```python
from build123d import *

# Parameters (mm, degrees)
BOX044_W          = 50
BOX044_H          = 20
BOX044_DEPTH      = 30
BOX_W             = 10
BOX_H             = 10
BOX_DEPTH         = 30
CYLINDER011_R     = 2
CYLINDER011_DEPTH = 24
CYLINDER009_R     = 2
CYLINDER009_DEPTH = 24
CYLINDER008_R     = 2
CYLINDER008_DEPTH = 24
BOX001_W          = 20
BOX001_H          = 33
BOX001_DEPTH      = 3


with BuildPart() as cube040:
    # Box044 → Box044 (new body)
    with BuildSketch(Plane(origin=(-25, -32, -1), x_dir=(1, 0, 0), z_dir=(0, 0, 1))):
        with Locations((25, 10)):
            Rectangle(BOX044_W, BOX044_H)
    extrude(amount=BOX044_DEPTH)


with BuildPart() as cube:
    # Box → Box (new body)
    with BuildSketch(Plane(origin=(-5, 2, -1), x_dir=(1, 0, 0), z_dir=(0, 0, 1))):
        with Locations((5, 5)):
            Rectangle(BOX_W, BOX_H)
    extrude(amount=BOX_DEPTH)


with BuildPart() as cylinder007:
    # Cylinder011 → Cylinder011 (new body)
    with BuildSketch(Plane(origin=(-10, -13, 4.3), x_dir=(0, 0, -1), z_dir=(1, 0, 0))):
        Circle(CYLINDER011_R)
    extrude(amount=CYLINDER011_DEPTH)


with BuildPart() as cylinder005:
    # Cylinder009 → Cylinder009 (new body)
    with BuildSketch(Plane(origin=(-10, -11, -1.3), x_dir=(0, 0, -1), z_dir=(1, 0, 0))):
        Circle(CYLINDER009_R)
    extrude(amount=CYLINDER009_DEPTH)


with BuildPart() as cylinder004:
    # Cylinder008 → Cylinder008 (new body)
    with BuildSketch(Plane(origin=(-10, 11, -1.3), x_dir=(0, 0, -1), z_dir=(1, 0, 0))):
        Circle(CYLINDER008_R)
    extrude(amount=CYLINDER008_DEPTH)


with BuildPart() as paste_extruder_charger:
    # Box001 → Box001 (new body)
    with BuildSketch(Plane(origin=(-8.25, -16.5, 0), x_dir=(1, 0, 0), z_dir=(0, 0, 1))):
        with Locations((10, 16.5)):
            Rectangle(BOX001_W, BOX001_H)
    extrude(amount=BOX001_DEPTH)

    # Cut001: cut Cylinder004
    add(cylinder004.part, mode=Mode.SUBTRACT)

    # Cut002: cut Cylinder005
    add(cylinder005.part, mode=Mode.SUBTRACT)

    # Cut003: cut Cylinder007
    add(cylinder007.part, mode=Mode.SUBTRACT)

    # Cut063: cut Cube
    add(cube.part, mode=Mode.SUBTRACT)

    # Cut062: cut Cube040
    add(cube040.part, mode=Mode.SUBTRACT)


with BuildPart() as paste_extruder_charger_1:
    # Cut062 placement: moved
    add(paste_extruder_charger.part.moved(Location((0, 58, 0))))


solid = paste_extruder_charger_1.part
```
For this review, take the finished solid that the model builds, in its own axes (mm). A direction names the side the tool comes from. Round coordinates to 2 decimals unless told otherwise and drop trailing zeros. Write each loop counter-clockwise with the first axis right and the second up, starting at its lowest first coordinate (ties: lowest second). Pieces come first, ordered by that corner, then holes. Notation, with made-up numbers: (88.5, 3) -> (113.5, 3) arc R23 ccw to (113.5, 12) -> close; hole circle Ø5 at (66, 26). An arc over 180 degrees is marked (long way). Use one line per item in the form item = value.
1) Mouldability with a two-part tool opening along X and no side actions: class faces 1 (the flat face through (2, 74.5, 1)), 2 (the flat face through (11.75, 60, 1)), 3 (the flat face through (-5, 65, 1)) as +X half, -X half, draft (parallel to the pull), parting line (faces both ways), or undercut.
Found:
face_1 = draft
face_2 = +X half
face_3 = undercut
2) Take a section at A-A, the plane x = 1. Write out the cut boundary in (y, z), and give its area (3 significant figures).
Found:
outline = (46, 0.43) arc R2 cw to (48.52, 0) -> (60, 0) -> (60, 3) -> (46.52, 3) arc R2 cw to (46, 2.57) -> close; (70, 0.43) arc R2 cw to (70.52, 0) -> (74.5, 0) -> (74.5, 3) -> (70, 3) -> close
area = 53.9 mm2
3) To check wall thickness, follow L1, parallel to Y at x = 3.5, z = 0.8; L2, parallel to X at y = 63, z = 0.95; L3, parallel to Y at x = 3, z = 2.6. State the ranges of each line that lie inside material, in increasing order. Write a range as from..to.
Found:
L1 = 46..60, 70..74.5
L2 = -8.25..-5, 5..11.75
L3 = 46.05..60, 70..74.5
4) Take a section at B-B, the plane y = 60.5. Write out the cut boundary in (x, z).
Found:
outline = (-8.25, 0) -> (-5, 0) -> (-5, 3) -> (-8.25, 3) -> close; (5, 0) -> (11.75, 0) -> (11.75, 3) -> (5, 3) -> close
5) Take a section at D-D, the plane x = 7.5. Write out the cut boundary in (y, z), and give its area (3 significant figures).
Found:
outline = (46, 0.43) arc R2 cw to (48.52, 0) -> (67.48, 0) arc R2 cw to (70.52, 0) -> (74.5, 0) -> (74.5, 3) -> (46.52, 3) arc R2 cw to (46, 2.57) -> close
area = 82.5 mm2
6) Tool access review of faces 4 (the cylindrical face through (1.61, 47.357, 0.668)), 5 (the flat face through (5, 65, 1)): name each direction out of +Z, -Z, +X, -X, +Y, -Y from which nothing blocks a thin tool from reaching the whole face with its end or side.
Found:
face_4 = -Z, +X, -X
face_5 = +Z, -Z
7) Take a section at C-C, the plane z = 1.8. Write out the cut boundary in (x, y).
Found:
outline = (-8.25, 46) -> (11.75, 46) -> (11.75, 74.5) -> (-8.25, 74.5) -> close; hole (-5, 60) -> (5, 60) -> (5, 70) -> (-5, 70) -> close
